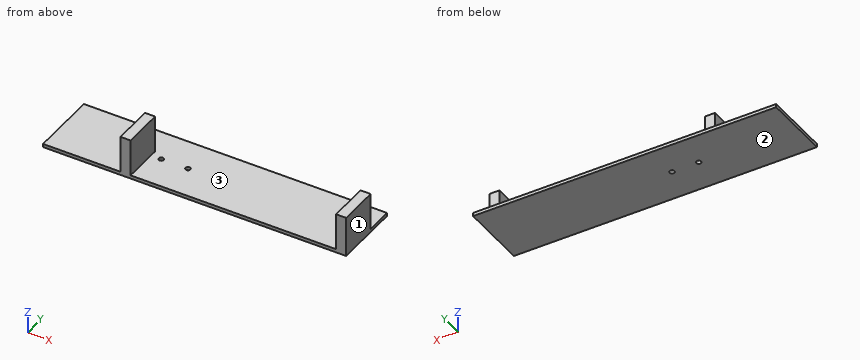
from build123d import *

# Parameters (mm, degrees)
SKETCH1_W               = 450
SKETCH1_H               = 100
BOSS_EXTRUDE1_DEPTH     = 5
SKETCH2_W               = 15
SKETCH2_H               = 60
BOSS_EXTRUDE2_DEPTH     = 55
SKETCH3_R               = 3.6
CUT_EXTRUDE1_DEPTH      = 56
CUT_EXTRUDE1_DEPTH_BACK = 6


with BuildPart() as part:
    # Sketch1 → Boss-Extrude1 (new body)
    with BuildSketch(Plane.XY):
        Rectangle(SKETCH1_W, SKETCH1_H)
    extrude(amount=BOSS_EXTRUDE1_DEPTH)

    # Sketch2 → Boss-Extrude2 (add)
    with BuildSketch(Plane.XY.offset(5)):
        with Locations((217.5, -20)):
            Rectangle(SKETCH2_W, SKETCH2_H)
        with Locations((-102.5, -20)):
            Rectangle(SKETCH2_W, SKETCH2_H)
    extrude(amount=BOSS_EXTRUDE2_DEPTH)

    # Sketch3 → Cut-Extrude1 (cut, two sides)
    with BuildSketch(Plane.XY.offset(5)) as cut_extrude1_sk:
        with Locations((-79.85, 0)):
            Circle(SKETCH3_R)
        with Locations((-40.15, 0)):
            Circle(SKETCH3_R)
    extrude(amount=CUT_EXTRUDE1_DEPTH, mode=Mode.SUBTRACT)
    extrude(cut_extrude1_sk.sketch, amount=-CUT_EXTRUDE1_DEPTH_BACK, mode=Mode.SUBTRACT)


solid = part.part
Work out the finished part from the listing and answer in its coordinate system (mm). Face numbers are marked on the shaded views. Round coordinates to 2 decimals unless told otherwise and drop trailing zeros. Loops run counter-clockwise (first coordinate to the right, second up) from the corner with the lowest first, then second, coordinate; pieces in that order, holes last. Notation, with made-up numbers: (-39, -2.5) -> (-21, -2.5) arc R6 ccw to (-21, 2.5) -> close; hole circle Ø3 at (80.25, -6). An arc over 180 degrees is marked (long way). Use one line per item in the form item = value.
(1) For a pull along X with two mould halves and no side action, classify the marked faces 1, 2 and 3 as released by +X, released by -X, zero draft, split by the parting line, or undercut.
Answer list:
face_1 = released by +X
face_2 = zero draft
face_3 = undercut
(2) Find section C-C on x = -120. Give the vertices of the cut face in (y, z), then the cut area to 3 significant figures.
Answer list:
outline = (-50, 0) -> (50, 0) -> (50, 5) -> (-50, 5) -> close
area = 500 mm2
(3) Flat-ended cylindrical pins translate along their axes: P1, Ø1.5, axis at y = -13.5, z = 34, coming from the -X side; P2, Ø10, axis at x = -39, y = -21, coming from the +Z side; P3, Ø16.5, axis at x = 214.5, z = 23, coming from the +Y side. Find the tip coordinate at first contact, or state that the pin passes through.
Answer list:
P1 = -110
P2 = 5
P3 = 10
(4) Find section D-D on y = 29. Give the vertices of the cut face in (x, z), then the cut area to 3 significant figures.
Answer list:
outline = (-225, 0) -> (225, 0) -> (225, 5) -> (-225, 5) -> close
area = 2,250 mm2
(5) Find section B-B on y = -35.5. Give the vertices of the cut face in (x, z).
Answer list:
outline = (-225, 0) -> (225, 0) -> (225, 60) -> (210, 60) -> (210, 5) -> (-95, 5) -> (-95, 60) -> (-110, 60) -> (-110, 5) -> (-225, 5) -> close
(6) Find section A-A on z = 37. Give the vertices of the cut face in (x, y).
Answer list:
outline = (-110, -50) -> (-95, -50) -> (-95, 10) -> (-110, 10) -> close; (210, -50) -> (225, -50) -> (225, 10) -> (210, 10) -> close
(7) Straight lines are drawn through the part: line 1 (Y direction, x = -40.15, z = 2.4); line 2 (X direction, y = -32, z = 15.5); line 3 (Z direction, x = 137.5, y = 43). For each, find the intervals that lie inside material, in ascending order.
Answer list:
line_1 = -50 to -3.6, 3.6 to 50
line_2 = -110 to -95, 210 to 225
line_3 = 0 to 5
